from build123d import *

# Parameters (mm, degrees)
SKETCH021_R          = 33
PAD017_DEPTH         = 37
PAD017_DEPTH_BACK    = 22.5
POCKET017_DEPTH      = 8.5
POCKET017_DEPTH_BACK = 13
SKETCH_2_R           = 6
POCKET018_DEPTH      = 50
POCKET018_DEPTH_BACK = 50
SKETCH028_R          = 6
POCKET019_DEPTH      = 180.001
POCKET020_START      = 10.5
SKETCH034_W          = 315.852005
SKETCH034_H          = 131
POCKET020_DEPTH      = 14.5


with BuildPart() as part:
    # Sketch021 → Pad017 (new body, two sides)
    with BuildSketch(Plane.XY) as pad017_sk:
        with BuildLine():
            Line((-110, -105), (110, -105))
            Line((110, -105), (120.90162, -105))
            ThreePointArc((120.90162, -105), (127.335146, -102.335146), (130, -95.90162))
            Line((130, -95.90162), (130, -89.09838))
            ThreePointArc((130, -89.09838), (127.335146, -82.664854), (120.90162, -80))
            Line((120.90162, -80), (119.09838, -80))
            ThreePointArc((110, -70.90162), (112.664854, -77.335146), (119.09838, -80))
            Line((110, -70.90162), (110, 0))
            Line((110, 70.90162), (110, 0))
            ThreePointArc((119.09838, 80), (112.664854, 77.335146), (110, 70.90162))
            Line((120.90162, 80), (119.09838, 80))
            ThreePointArc((120.90162, 80), (127.335146, 82.664854), (130, 89.09838))
            Line((130, 95.90162), (130, 89.09838))
            ThreePointArc((130, 95.90162), (127.335146, 102.335146), (120.90162, 105))
            Line((110, 105), (120.90162, 105))
            Line((110, 105), (-110, 105))
            Line((-110, 105), (-110, 0))
            Line((-110, -105), (-110, 0))
        make_face()
        Circle(SKETCH021_R, mode=Mode.SUBTRACT)
    extrude(amount=-PAD017_DEPTH)
    extrude(pad017_sk.sketch, amount=PAD017_DEPTH_BACK)

    # Sketch_1 → Pocket017 (cut, two sides)
    with BuildSketch(Plane.XY) as pocket017_sk:
        Polygon((145.597992, 65.5), (0, 65.5), (-153.015656, 65.5), (-153.015656, -65.5), (0, -65.5), (145.597992, -65.5), align=None)
    extrude(amount=-POCKET017_DEPTH, mode=Mode.SUBTRACT)
    extrude(pocket017_sk.sketch, amount=POCKET017_DEPTH_BACK, mode=Mode.SUBTRACT)

    # Sketch_2 → Pocket018 (cut, two sides)
    with BuildSketch(Plane.XY) as pocket018_sk:
        with Locations((-118, 93)):
            Circle(SKETCH_2_R)
        with Locations((118, 93)):
            Circle(SKETCH_2_R)
        with Locations((-118, -93)):
            Circle(SKETCH_2_R)
        with Locations((118, -93)):
            Circle(SKETCH_2_R)
        Polygon((-0.25, 33.607407), (-0.25, 47.5), (126.736248, 47.5), (126.736248, 47), (0.25, 47), (0.25, 33.607407), align=None)
        with BuildLine():
            ThreePointArc((86.75, 75), (87.81066, 75.43934), (88.25, 76.5))
            Line((88.25, 105), (88.25, 76.5))
            Line((88.25, 105), (6.75, 105))
            Line((6.75, 105), (6.75, 76.5))
            ThreePointArc((6.75, 76.5), (7.18934, 75.43934), (8.25, 75))
            Line((86.75, 75), (8.25, 75))
        make_face()
        Polygon((-0.067348, -33.607407), (-0.067348, -47.5), (126.736248, -47.5), (126.736248, -47), (0.25, -47), (0.25, -33.607407), align=None)
        with BuildLine():
            ThreePointArc((-88.25, 76.5), (-87.81066, 75.43934), (-86.75, 75))
            Line((-86.75, 75), (-8.25, 75))
            ThreePointArc((-8.25, 75), (-7.18934, 75.43934), (-6.75, 76.5))
            Line((-6.75, 105), (-6.75, 76.5))
            Line((-88.25, 105), (-6.75, 105))
            Line((-88.25, 105), (-88.25, 76.5))
        make_face()
        with BuildLine():
            ThreePointArc((88.25, -76.5), (87.81066, -75.43934), (86.75, -75))
            Line((86.75, -75), (8.25, -75))
            ThreePointArc((8.25, -75), (7.18934, -75.43934), (6.75, -76.5))
            Line((6.75, -105), (6.75, -76.5))
            Line((88.25, -105), (6.75, -105))
            Line((88.25, -105), (88.25, -76.5))
        make_face()
        with BuildLine():
            ThreePointArc((-86.75, -75), (-87.81066, -75.43934), (-88.25, -76.5))
            Line((-88.25, -105), (-88.25, -76.5))
            Line((-88.25, -105), (-6.75, -105))
            Line((-6.75, -105), (-6.75, -76.5))
            ThreePointArc((-6.75, -76.5), (-7.18934, -75.43934), (-8.25, -75))
            Line((-86.75, -75), (-8.25, -75))
        make_face()
    extrude(amount=-POCKET018_DEPTH, mode=Mode.SUBTRACT)
    extrude(pocket018_sk.sketch, amount=POCKET018_DEPTH_BACK, mode=Mode.SUBTRACT)

    # Sketch028 → Pocket019 (cut, through all)
    with BuildSketch(Plane.XZ.offset(75)):
        with Locations((74, -21.75)):
            Circle(SKETCH028_R)
    extrude(amount=-POCKET019_DEPTH, mode=Mode.SUBTRACT)

    # Sketch034 → Pocket020 (cut)
    with BuildSketch(Plane.XY.offset(POCKET020_START)):
        with Locations((3.702202, 0)):
            Rectangle(SKETCH034_W, SKETCH034_H)
    extrude(amount=POCKET020_DEPTH, mode=Mode.SUBTRACT)


solid = part.part
For this review, take the finished solid that the model builds, in its own axes (mm). A direction names the side the tool comes from. Round coordinates to 2 decimals unless told otherwise and drop trailing zeros. Order: outer loops, then holes, each group sorted by start corner. A loop starts at its lowest first (then second) coordinate and runs counter-clockwise, first axis right, second up. Notation, with made-up numbers: (81, 12.5) -> (135, 12.5) arc R38 ccw to (135, 51.5) -> close; hole circle Ø3 at (-27, 86). An arc over 180 degrees is marked (long way). Put each result on its own line as item: value.
Q1. Add section D-D on x = 36. Write out the cut boundary in (y, z).
Check result:
outline: (-75, -37) -> (-47.5, -37) -> (-47.5, -8.5) -> (-65.5, -8.5) -> (-65.5, 22.5) -> (-75, 22.5) -> close; (-47, -37) -> (47, -37) -> (47, -8.5) -> (-47, -8.5) -> close; (47.5, -37) -> (75, -37) -> (75, 22.5) -> (65.5, 22.5) -> (65.5, -8.5) -> (47.5, -8.5) -> close
Q2. Add section C-C on y = 28. Write out the cut boundary in (x, z), plus the area to 3 significant figures.
Check result:
outline: (-110, -37) -> (-17.46, -37) -> (-17.46, -8.5) -> (-110, -8.5) -> close; (17.46, -37) -> (110, -37) -> (110, -8.5) -> (17.46, -8.5) -> close; hole circle Ø12 at (74, -21.75)
area: 5,160 mm2
Q3. Mouldability with a two-part tool opening along X and no side actions: class faces 1 (the flat face through (110, 62, -21)), 2 (the flat face through (48, -75, -7)), 3 (the flat face through (0, -105, -8)) as pulls with the +X half, pulls with the -X half, needs draft (parallel to the pull), parting line crosses it, or undercut.
Check result:
face 1: pulls with the +X half
face 2: undercut
face 3: needs draft
Q4. Machinability: for faces 4 (the flat face through (6.75, -91, -7)), 5 (the flat face through (-2, -65.5, 7)), 6 (the flat face through (56, -47, -23)), which of the approach directions +Z, -Z, +X, -X, +Y, -Y give a long, thin tool a straight path to every point of the face, cutting with its end or side? Answer none if there is none.
Check result:
face 4: +Z, -Z, -Y
face 5: +Z, +X, -X
face 6: +Z, -Z, +X
Q5. For probe 1 along Y at (x, z) = (67, -28.5); probe 2 along Y at (x, z) = (91, -30.5); probe 3 along Z at (x, y) = (74, -27), list the stretches that pass through material, from the lowest coordinate up. Write a range as [from, to].
Check result:
probe 1: [-75, -47.5], [-47, 47], [47.5, 75]
probe 2: [-105, -47.5], [-47, 47], [47.5, 105]
probe 3: [-37, -27.75], [-15.75, -8.5]
Q6. Add section B-B on x = 74. Write out the cut boundary in (y, z), plus the area to 3 significant figures.
Check result:
outline: (-75, -37) -> (-47.5, -37) -> (-47.5, -27.75) -> (-75, -27.75) -> close; (-75, -15.75) -> (-47.5, -15.75) -> (-47.5, -8.5) -> (-65.5, -8.5) -> (-65.5, 22.5) -> (-75, 22.5) -> close; (-47, -37) -> (47, -37) -> (47, -27.75) -> (-47, -27.75) -> close; (-47, -15.75) -> (47, -15.75) -> (47, -8.5) -> (-47, -8.5) -> close; (47.5, -37) -> (75, -37) -> (75, -27.75) -> (47.5, -27.75) -> close; (47.5, -15.75) -> (75, -15.75) -> (75, 22.5) -> (65.5, 22.5) -> (65.5, -8.5) -> (47.5, -8.5) -> close
area: 3,050 mm2
Q7. Insertion check: pin 1 Ø19 at (x, z) = (74, -21.75) entering from -Y; pin 2 Ø10 at (x, y) = (-2, 58) entering from +Z; pin 3 Ø6 at (x, z) = (35.5, -4) entering from +Y. Each pin has a flat end and moves straight along its axis. Give the tip position at first contact, or say it passes through.
Check result:
pin 1: y = -75
pin 2: z = -8.5
pin 3: y = 75
Q8. Add section A-A on y = 93. Write out the cut boundary in (x, z).
Check result:
outline: (-110, -37) -> (-88.25, -37) -> (-88.25, 22.5) -> (-110, 22.5) -> close; (-6.75, -37) -> (6.75, -37) -> (6.75, 22.5) -> (-6.75, 22.5) -> close; (88.25, -37) -> (112, -37) -> (112, 22.5) -> (88.25, 22.5) -> close; (124, -37) -> (130, -37) -> (130, 22.5) -> (124, 22.5) -> close
